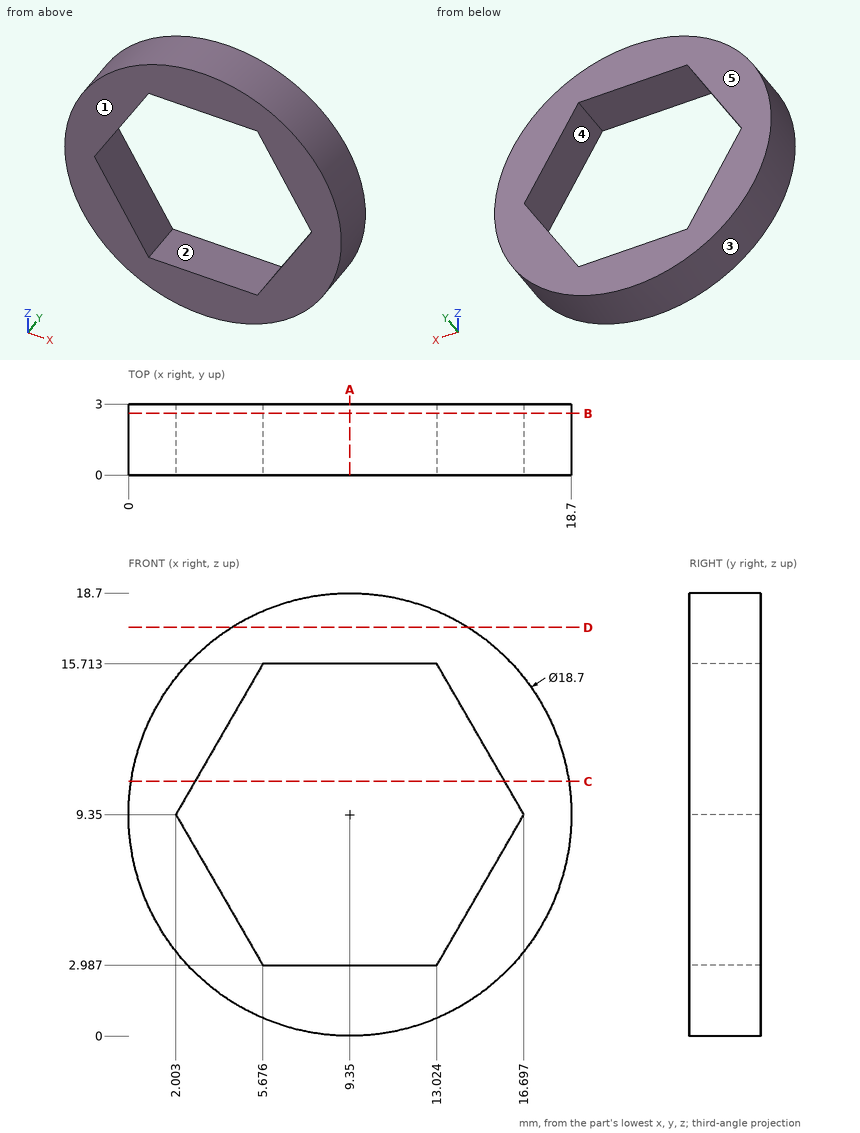
Check sheet for the drawn part. Datum: minimum x, y, z corner. Units: mm. A direction names the side the tool comes from. Round coordinates to 2 decimals unless told otherwise and drop trailing zeros. Write each loop counter-clockwise with the first axis right and the second up, starting at its lowest first coordinate (ties: lowest second). Pieces come first, ordered by that corner, then holes. Notation, with made-up numbers: (43, -2) - (63, -2) arc R17 ccw to (63, 18) - close; hole circle Ø6 at (58.25, 52). An arc over 180 degrees is marked (long way). Return JSON: item names as keys, results as strings.
Q1. Scan lines: L1, parallel to X at y = 2.75, z = 10.25 (1 decimal); L2, parallel to Z at x = 9.25, y = 2; L3, parallel to Z at x = 12.25, y = 2.7. Record each from-to range of solid material in increasing order. Write a range as from..to.
Returned:
{"L1": "x = 0..2.5, 16.2..18.7", "L2": "z = 0..2.99, 15.71..18.7", "L3": "z = 0.46..2.99, 15.71..18.24"}
Q2. Cross-section at B-B (y = 2.6). Record the boundary of the cut face in (x, z).
Returned:
{"outline": "circle Ø18.7 at (9.35, 9.35); hole (2, 9.35) - (5.68, 2.99) - (13.02, 2.99) - (16.7, 9.35) - (13.02, 15.71) - (5.68, 15.71) - close"}
Q3. Draft check along Z on the marked faces 3, 4 and 5. Enter one of: released by +Z, released by -Z, zero draft, split by the parting line, or undercut.
Returned:
{"face 3": "split by the parting line", "face 4": "undercut", "face 5": "zero draft"}
Q4. Cross-section at C-C (z = 10.75). Record the boundary of the cut face in (x, y) (1 decimal).
Returned:
{"outline": "(0.1, 0) - (2.8, 0) - (2.8, 3) - (0.1, 3) - close; (15.9, 0) - (18.6, 0) - (18.6, 3) - (15.9, 3) - close"}
Q5. Access from +Z, -Z, +X, -X, +Y, -Y to the whole of each face (thin tool, end or side, straight path). Record for the marked faces 1 and 2.
Returned:
{"face 1": "+Z, -Z, +X, -X, -Y", "face 2": "+Y, -Y"}
Q6. Depth check by flat-ended pin: P1, Ø1, axis at y = 2.5, z = 3.5, coming from the -X side; P2, Ø1.5, axis at y = 2.5, z = 13.5, coming from the -X side; P3, Ø0.9, axis at x = 9, y = 2, coming from the +Z side; P4, Ø1.5, axis at x = 11.5, y = 1.5, coming from the -Z side (1 decimal). Enter the tip coordinate at first touch or a pass-through.
Returned:
{"P1": "stops at x = 1.68", "P2": "stops at x = 0.64", "P3": "stops at z = 18.7", "P4": "stops at z = 0.1"}
Q7. Cross-section at D-D (z = 17.25). Record the boundary of the cut face in (x, y).
Returned:
{"outline": "(4.35, 0) - (14.35, 0) - (14.35, 3) - (4.35, 3) - close"}
Q8. Cross-section at A-A (x = 9.35). Record the boundary of the cut face in (y, z), then the cut area to 3 significant figures.
Returned:
{"outline": "(0, 0) - (3, 0) - (3, 2.99) - (0, 2.99) - close; (0, 15.71) - (3, 15.71) - (3, 18.7) - (0, 18.7) - close", "area": "17.9 mm²"}
